Design review of the part built by this model. Coordinates are the model's own, in mm. Face numbers are marked on the shaded views. A direction names the side the tool comes from. Round coordinates to 2 decimals unless told otherwise and drop trailing zeros. Order: outer loops, then holes, each group sorted by start corner. A loop starts at its lowest first (then second) coordinate and runs counter-clockwise, first axis right, second up. Notation, with made-up numbers: (35, 88.25) - (47, 88.25) arc R22 ccw to (47, 119.25) - close; hole circle Ø11 at (54.5, 53.25). An arc over 180 degrees is marked (long way). Write item = value, one per line.
from build123d import *

# Parameters (mm, degrees)
SKETCH_1_W          = 100
SKETCH_1_H          = 100
SKETCH_1_W_2        = 94
SKETCH_1_H_2        = 94
EXTRUDE_1_DEPTH     = 50
EXTRUDE_2_REACH     = 122.037
SKETCH_4_W          = 66
SKETCH_4_H          = 3
SKETCH_2_R          = 2.5
CUT_EXTRUDE_1_DEPTH = 50
SKETCH_9_R          = 2.5
CUT_EXTRUDE_5_DEPTH = 123.474487139
SKETCH_10_R         = 2.5
CUT_EXTRUDE_6_DEPTH = 20


with BuildPart() as part:
    # 草圖1 → 填料-伸長1 (new, symmetric)
    with BuildSketch(Plane.XY):
        Rectangle(SKETCH_1_W, SKETCH_1_H)
        Rectangle(SKETCH_1_W_2, SKETCH_1_H_2, mode=Mode.SUBTRACT)
    extrude(amount=EXTRUDE_1_DEPTH, both=True)

    # 草圖4 → 填料-伸長2 (add, up to next)
    with BuildSketch(Plane(origin=(-47, 0, 0), x_dir=(0, 0, -1), z_dir=(1, 0, 0)), mode=Mode.PRIVATE) as extrude_2_sk1:
        with Locations((0, 38.5)):
            Rectangle(SKETCH_4_W, SKETCH_4_H)
    extrude_2_tool1 = extrude(extrude_2_sk1.sketch, amount=EXTRUDE_2_REACH, mode=Mode.PRIVATE) - part.part
    add(extrude_2_tool1.solids().sort_by_distance((-47, 38.5, 0))[0])

    # 草圖2 → 除料-伸長1 (cut, symmetric)
    with BuildSketch(Plane(origin=(0, 0, 0), x_dir=(0, 0, -1), z_dir=(1, 0, 0))):
        Circle(SKETCH_2_R)
    extrude(amount=CUT_EXTRUDE_1_DEPTH, both=True, mode=Mode.SUBTRACT)

    # 草圖9 → 除料-伸長5 (cut, through all)
    with BuildSketch(Plane(origin=(0, 50, 0), x_dir=(1, 0, 0), z_dir=(0, 1, 0))):
        with Locations(Location((-30, 20, 0), (0, 0, 270))):
            Circle(SKETCH_9_R)
        with Locations(Location((30, 20, 0), (0, 0, 270))):
            Circle(SKETCH_9_R)
    extrude(amount=-CUT_EXTRUDE_5_DEPTH, mode=Mode.SUBTRACT)

    # 草圖10 → 除料-伸長6 (cut)
    with BuildSketch(Plane(origin=(0, 40, 0), x_dir=(1, 0, 0), z_dir=(0, 1, 0))):
        with Locations(Location((-30, 0, 0), (0, 0, 270))):
            Circle(SKETCH_10_R)
        with Locations(Location((30, 0, 0), (0, 0, 270))):
            Circle(SKETCH_10_R)
    extrude(amount=-CUT_EXTRUDE_6_DEPTH, mode=Mode.SUBTRACT)


solid = part.part
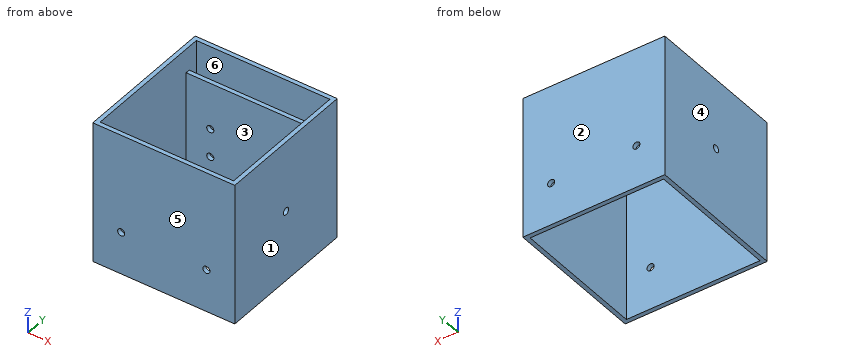
Item 1: The part is to be moulded in two halves that separate along X. For the marked faces 1, 2, 3 and 4, say which applies: +X half, -X half, draft (parallel to the pull), parting line (faces both ways), or undercut.
Data:
face_1 = +X half
face_2 = draft
face_3 = undercut
face_4 = -X half
Item 2: For line 1 along X through (y, z) = (37.8, 0); line 2 along Y through (x, z) = (2.5, -1.5); line 3 along Y through (x, z) = (-48.8, 0), list the stretches that pass through material, from the lowest coordinate up. Write a range as [from, to].
Data:
line_1 = [-50, -32.5], [-27.5, 27.5], [32.5, 50]
line_2 = [-50, -47], [37, 40], [47, 50]
line_3 = [-50, -2.5], [2.5, 50]
Item 3: For the marked faces 5 and 6, list the 3-axis set-ups (+Z, -Z, +X, -X, +Y, -Y) from which the entire face can be reached by the end or side of a thin tool; tool diameter is ignored.
Data:
face_5 = +Z, -Z, +X, -X, -Y
face_6 = +Z, -Z
Item 4: Take a section at A-A, the plane z = 0. State the section outline as (x, y) points.
Data:
outline = (-50, -50) - (50, -50) - (50, -2.5) - (47, -2.5) - (47, -47) - (-47, -47) - (-47, -2.5) - (-50, -2.5) - close; (-50, 2.5) - (-47, 2.5) - (-47, 37) - (-32.5, 37) - (-32.5, 40) - (-47, 40) - (-47, 47) - (47, 47) - (47, 40) - (32.5, 40) - (32.5, 37) - (47, 37) - (47, 2.5) - (50, 2.5) - (50, 50) - (-50, 50) - close; (-27.5, 37) - (27.5, 37) - (27.5, 40) - (-27.5, 40) - close
Item 5: Take a section at D-D, the plane y = 0. State the section outline as (x, z) points.
Data:
outline = (-50, -50) - (-47, -50) - (-47, -2.5) - (-50, -2.5) - close; (-50, 2.5) - (-47, 2.5) - (-47, 50) - (-50, 50) - close; (47, -50) - (50, -50) - (50, -2.5) - (47, -2.5) - close; (47, 2.5) - (50, 2.5) - (50, 50) - (47, 50) - close
Item 6: Take a section at C-C, the plane x = -34.5. State the section outline as (y, z) points, and give its area (3 significant figures).
Data:
outline = (-50, -50) - (-47, -50) - (-47, 50) - (-50, 50) - close; (37, -33) - (40, -33) - (40, 33) - (37, 33) - close; (47, -50) - (50, -50) - (50, 50) - (47, 50) - close
area = 798 mm2
Item 7: Take a section at B-B, the plane y = 27.5. State the section outline as (x, z) points, and give its area (3 significant figures).
Data:
outline = (-50, -50) - (-47, -50) - (-47, 50) - (-50, 50) - close; (47, -50) - (50, -50) - (50, 50) - (47, 50) - close
area = 600 mm2
Item 8: Insertion check: P1, Ø6.5, axis at x = 30, z = -20, coming from the +Y side; P2, Ø4, axis at x = -30, z = -20, coming from the +Y side; P3, Ø0.9, axis at x = -17, y = 38.5, coming from the +Z side; P4, Ø2.5, axis at x = 10, y = 38.5, coming from the -Z side. Each pin has a flat end and moves straight along its axis. Give the tip position at first contact, or say it passes through.
Data:
P1 = 50
P2 = through
P3 = 33
P4 = -33
